Build history of the part. All positions in model axes, mm. Face numbers are marked on the shaded views. A direction names the side the tool comes from. Give positions to 0.01 mm unless a question says otherwise; leave off trailing zeros. Loops run counter-clockwise (first coordinate to the right, second up) from the corner with the lowest first, then second, coordinate; pieces in that order, holes last.
1) 3-axis set-ups, long thin cutter, end or side, ignore diameter. For the marked faces 1, 2, 3 and 4: which of +Z, -Z, +X, -X, +Y, -Y reach the whole face in a straight line?
2) Band-saw the part on D-D on x = 3. List the corners of the cut face in (y, z), then the cut area to 3 significant figures.
3) Flat gauge pins, fed straight in: P1, Ø3, axis at x = 10, y = 3, coming from the -Z side; P2, Ø1.5, axis at x = 6, z = 2, coming from the -Y side; P3, Ø1, axis at x = 10.5, z = 1, coming from the +Y side; P4, Ø1, axis at x = 9.5, z = 0.5, coming from the -Y side. Where does each tip first touch, or does it go through?
4) Band-saw the part on C-C on y = 1.9. List the corners of the cut face in (x, z).
5) Two-plate mould, pull along Z, no slides. Class the marked faces 5, 6 and 7: +Z half, -Z half, draft (parallel to the pull), parting line (faces both ways), or undercut.
6) Band-saw the part on B-B on y = 3.25. List the corners of the cut face in (x, z), then the cut area to 3 significant figures.
7) Wall check: line 1 (Y direction, x = 10.8, z = 1.25); line 2 (Z direction, x = 4.5, y = 3.9); line 3 (Z direction, x = 8.85, y = 2.8). Give the ranges that are in metal, low to high.
```python
from build123d import *

# Parameters (mm, degrees)
F1_DEPTH = 0.55
F2_W     = 4.5
F2_H     = 2.5
F3_DEPTH = 1.95
F4_R     = 1.24999
F5_R     = 0.7
F6_DEPTH = 25


# Not quite as in the source:
# - a fillet or chamfer is up to 0.001 mm smaller than in the source, because OpenCascade refuses the exact size


with BuildPart() as f1:
    # F0 (on Top) → F1 (new body)
    with BuildSketch(Plane.XY):
        with BuildLine():
            Line((7.1757397782, 1.55), (12, 1.55))
            Line((12, 1.55), (12, 4.05))
            Line((12, 4.05), (7.1757397782, 4.05))
            ThreePointArc((7.1757397782, 4.05), (6.8353451552, 4.0707678217), (6.5, 4.1327632138))
            ThreePointArc((6.5, 4.1327632138), (6.1928359056, 4.2281876541), (5.8986420809, 4.3582091838))
            Line((5.8986420809, 4.3582091838), (4.0770976972, 5.2917908162))
            ThreePointArc((4.0770976972, 5.2917908162), (3.4568811592, 5.5218572965), (2.8, 5.6))
            Line((2.8, 5.6), (2.8, 4.65))
            ThreePointArc((2.8, 4.65), (4.1081475452, 4.1081475452), (4.65, 2.8))
            ThreePointArc((4.65, 2.8), (4.1081475452, 1.4918524548), (2.8, 0.95))
            Line((2.8, 0.95), (2.8, 0))
            ThreePointArc((2.8, 0), (3.4568811592, 0.0781427035), (4.0770976972, 0.3082091838))
            Line((4.0770976972, 0.3082091838), (5.8986420809, 1.2417908162))
            ThreePointArc((5.8986420809, 1.2417908162), (6.1928359056, 1.3718123459), (6.5, 1.4672367862))
            ThreePointArc((6.5, 1.4672367862), (6.8353451552, 1.5292321783), (7.1757397782, 1.55))
        make_face()
        with BuildLine():
            ThreePointArc((0, 2.8), (0.8201010127, 0.8201010127), (2.8, 0))
            Line((2.8, 0), (2.8, 0.95))
            ThreePointArc((2.8, 0.95), (0.95, 2.8), (2.8, 4.65))
            Line((2.8, 4.65), (2.8, 5.6))
            ThreePointArc((2.8, 5.6), (0.8201010127, 4.7798989873), (0, 2.8))
        make_face()
    extrude(amount=F1_DEPTH)

    # F2 (on face) → F3 (join)
    with BuildSketch(Plane.XY.offset(0.55)):
        with Locations((9.75, 2.8)):
            Rectangle(F2_W, F2_H)
    extrude(amount=F3_DEPTH)

    # F4 (radius 1.25 in the source; OpenCascade refuses exactly that, so slightly less here)
    f4_edges = [f1.edges().sort_by_distance(p)[0] for p in [
        (9.75, 4.05, 2.5),
        (9.75, 1.55, 2.5),
    ]]
    fillet(f4_edges, radius=F4_R)

    # F5 (on face) → F6 (cut)
    with BuildSketch(Plane.YZ.offset(12)):
        with Locations((2.8, 1.25)):
            Circle(F5_R)
    extrude(amount=-F6_DEPTH, mode=Mode.SUBTRACT)


solid = f1.part
```
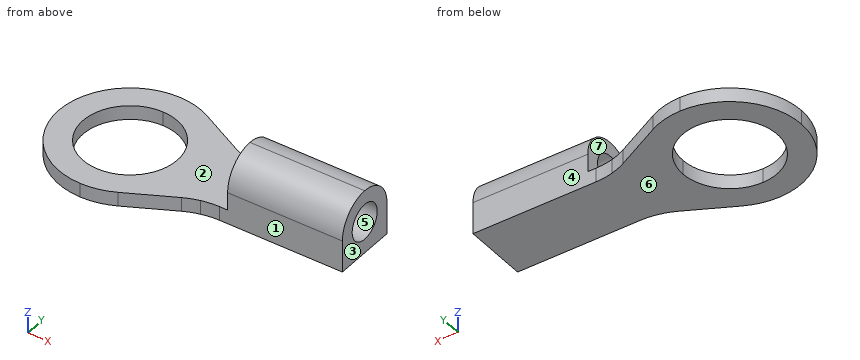
Findings below:
1. face 1: +Z, -Z, +X, -Y
1. face 2: +Z, -X, +Y, -Y
1. face 3: +Z, -Z, +X, +Y, -Y
1. face 4: +Z, -Z, +X, +Y
2. outline: (0.01, 0) - (0.96, 0) - (0.96, 0.55) - (0.01, 0.55) - close; (4.64, 0) - (5.59, 0) - (5.59, 0.55) - (4.64, 0.55) - close
2. area: 1.05 mm2
3. P1: stops at z = 0
3. P2: passes through
3. P3: stops at y = 4.05
3. P4: stops at y = 1.55
4. outline: (0.15, 0) - (1.18, 0) - (1.18, 0.55) - (0.15, 0.55) - close; (4.42, 0) - (12, 0) - (12, 2.12) - (7.5, 2.12) - (7.5, 0.55) - (4.42, 0.55) - close
5. face 5: undercut
5. face 6: -Z half
5. face 7: draft
6. outline: (0.04, 0) - (1.01, 0) - (1.01, 0.55) - (0.04, 0.55) - close; (4.59, 0) - (12, 0) - (12, 0.71) - (7.5, 0.71) - (7.5, 0.55) - (4.59, 0.55) - close; (7.5, 1.79) - (12, 1.79) - (12, 2.42) - (7.5, 2.42) - close
6. area: 8.18 mm2
7. line 1: y = 1.55 to 2.1, 3.5 to 4.05
7. line 2: z = 0 to 0.55
7. line 3: z = 0 to 0.55, 1.95 to 2.5
